from build123d import *

# Parameters (mm, degrees)
F0_R     = 30
F0_R_2   = 20
F1_DEPTH = 100
F3_DEPTH = 50
F5_DEPTH = 10


with BuildPart() as f1:
    # F0 (on Front) → F1 (new body)
    with BuildSketch(Plane.XZ):
        Circle(F0_R)
        Circle(F0_R_2, mode=Mode.SUBTRACT)
    extrude(amount=F1_DEPTH)

    # F2 (on Front) → F3 (join)
    with BuildSketch(Plane.XZ):
        with BuildLine():
            Line((-30.1086945207, 100), (-30.1086945207, 0))
            add(Edge.make_bspline(
                [(-30.1086945207, 0), (-28.1945433239, 8.0804869026), (-24.3908970229, 24.1373763311), (-0.0363134271, 33.4382771528), (25.4775085898, 23.5551805153), (28.4355133491, 7.7691491651), (29.8913054793, 0)],
                knots=[0, 0, 0, 0, 0.2515656937, 0.4998909813, 0.7538696409, 1, 1, 1, 1], degree=3))
            Line((29.8913054793, 0), (29.8913054793, 100))
            Line((29.8913054793, 100), (-30.1086945207, 100))
        make_face()
    extrude(amount=F3_DEPTH)

    # F4 (on Right) → F5 (join)
    with BuildSketch(Plane.YZ):
        Polygon((-99.8394265771, 30.9073068202), (-50.5473278463, 30.9073068202), (-49.9311797321, 51.420763135), align=None)
    extrude(amount=F5_DEPTH)


solid = f1.part
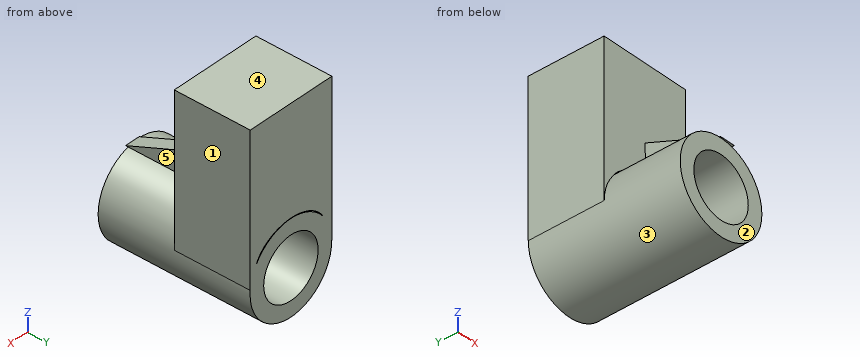
The model under review builds one solid part; all positions refer to its coordinate system, in mm. Face numbers are marked on the shaded views. A direction names the side the tool comes from. Round coordinates to 2 decimals unless told otherwise and drop trailing zeros. Order: outer loops, then holes, each group sorted by start corner. A loop starts at its lowest first (then second) coordinate and runs counter-clockwise, first axis right, second up. Notation, with made-up numbers: (48.5, -12.75) -> (72.5, -12.75) arc R20 ccw to (72.5, 24.25) -> close; hole circle Ø1 at (69, 10.25). An arc over 180 degrees is marked (long way). Write item = value, one per line. Start each with the question number.
Item 1: Consider section C-C on y = -57. Write out the cut boundary in (x, z), plus the area to 3 significant figures.
Item 2: For the marked faces 1 and 2, list the 3-axis set-ups (+Z, -Z, +X, -X, +Y, -Y) from which the entire face can be reached by the end or side of a thin tool; tool diameter is ignored.
Item 3: Consider section B-B on z = -3. Write out the cut boundary in (x, y), plus the area to 3 significant figures.
Item 4: For line 1 along Z through (x, y) = (0, -44); line 2 along Z through (x, y) = (-15.5, -20); line 3 along Y through (x, z) = (-7, 81), list the stretches that pass through material, from the lowest coordinate up.
Item 5: Consider section D-D on z = 27. Count the separate pieces of the cut face and the enclosed holes in it, plus the area to 3 significant figures.
Item 6: Consider section A-A on y = -81. Write out the cut boundary in (x, z), plus the area to 3 significant figures.
Item 7: Mouldability with a two-part tool opening along Z and no side actions: class the marked faces 3, 4 and 5 as released by +Z, released by -Z, zero draft, split by the parting line, or undercut.
Item 8: Clearance check with flat-ended pins moving along their axes: pin 1 Ø12 at (x, y) = (-17.5, -43.5) entering from -Z; pin 2 Ø8 at (x, y) = (3, -73) entering from -Z; pin 3 Ø3 at (x, y) = (-18, -75.5) entering from -Z; pin 4 Ø24 at (x, z) = (0, 0) entering from -Y. State where each tip first meets the part, or that it passes through.
Conclusion:
q1.outline = circle Ø60 at (0, 0); (0, 30.91) -> (10, 30.91) -> (10, 48.52) -> (0, 48.52) -> close; hole circle Ø40 at (0, 0)
q1.area = 1,750 mm2
q2.face_1 = +Z, +X, +Y, -Y
q2.face_2 = +Z, -Z, +X, -X, -Y
q3.outline = (-29.85, -100) -> (-19.77, -100) -> (-19.77, 0) -> (-29.85, 0) -> close; (19.77, -100) -> (29.85, -100) -> (29.85, 0) -> (19.77, 0) -> close
q3.area = 2,020 mm2
q4.line_1 = -30 to -20, 20 to 30, 30.23 to 100
q4.line_2 = -25.69 to -12.64, 12.64 to 25.69, 26.32 to 100
q4.line_3 = -50 to 0
q5.separate_pieces = 3
q5.enclosed_holes = 0
q5.area = 4,200 mm2
q6.outline = circle Ø60 at (0, 0); (0, 30.91) -> (10, 30.91) -> (10, 38.65) -> (0, 38.65) -> close; hole circle Ø40 at (0, 0)
q6.area = 1,650 mm2
q7.face_3 = undercut
q7.face_4 = released by +Z
q7.face_5 = zero draft
q8.pin_1 = -27.71
q8.pin_2 = -30
q8.pin_3 = -25.05
q8.pin_4 = through
